from build123d import *

# Parameters (mm, degrees)
F0_W     = 47.752
F0_H     = 16.1036
F1_DEPTH = 5.588
F2_R     = 2.413
F3_DEPTH = 1.8034
F5_W     = 45.212
F5_H     = 13.5636
F5_R     = 3.2512
F6_DEPTH = 9.906


with BuildPart() as f1:
    # F0 (on Top) → F1 (new body, symmetric)
    with BuildSketch(Plane.XY):
        Rectangle(F0_W, F0_H)
    extrude(amount=F1_DEPTH, both=True)

    # F2 (on face) → F3 (join)
    with BuildSketch(Plane.XY.offset(5.588)):
        with Locations((-19.9771, 4.1275)):
            Circle(F2_R)
        with Locations((-12.3571, 4.1275)):
            Circle(F2_R)
        with Locations((-4.7371, 4.1275)):
            Circle(F2_R)
        with Locations((2.8829, 4.1275)):
            Circle(F2_R)
        with Locations((10.5029, 4.1275)):
            Circle(F2_R)
        with Locations((-19.9771, -4.1275)):
            Circle(F2_R)
        with Locations((-12.3571, -4.1275)):
            Circle(F2_R)
        with Locations((-4.7371, -4.1275)):
            Circle(F2_R)
        with Locations((2.8829, -4.1275)):
            Circle(F2_R)
        with Locations((10.5029, -4.1275)):
            Circle(F2_R)
        with Locations((18.1229, 4.1275)):
            Circle(F2_R)
        with Locations((18.1229, -4.1275)):
            Circle(F2_R)
    extrude(amount=F3_DEPTH)

    # F5 (on face) → F6 (cut)
    with BuildSketch(Plane(origin=(0, 0, -5.588), x_dir=(1, 0, 0), z_dir=(0, 0, -1))):
        Rectangle(F5_W, F5_H)
        with Locations((-16.51, 0)):
            Circle(F5_R, mode=Mode.SUBTRACT)
        with Locations((-8.3058, 0)):
            Circle(F5_R, mode=Mode.SUBTRACT)
        with Locations((-0.1016, 0)):
            Circle(F5_R, mode=Mode.SUBTRACT)
        with Locations((8.1026, 0)):
            Circle(F5_R, mode=Mode.SUBTRACT)
        with Locations((16.3068, 0)):
            Circle(F5_R, mode=Mode.SUBTRACT)
    extrude(amount=-F6_DEPTH, mode=Mode.SUBTRACT)


solid = f1.part
Input: part model. Units: mm. Frame: model coordinates. A direction names the side the tool comes from. Coordinates: 2 decimals unless noted, no trailing zeros. Order: outer loops, then holes, each group sorted by start corner. A loop starts at its lowest first (then second) coordinate and runs counter-clockwise, first axis right, second up.
1. Cut plane B-B, the plane y = 0. Return loops of the section in (x, z).
Checked values:
outline: (-23.88, -5.59) - (-22.61, -5.59) - (-22.61, 4.32) - (-19.76, 4.32) - (-19.76, -5.59) - (-13.26, -5.59) - (-13.26, 4.32) - (-11.56, 4.32) - (-11.56, -5.59) - (-5.05, -5.59) - (-5.05, 4.32) - (-3.35, 4.32) - (-3.35, -5.59) - (3.15, -5.59) - (3.15, 4.32) - (4.85, 4.32) - (4.85, -5.59) - (11.35, -5.59) - (11.35, 4.32) - (13.06, 4.32) - (13.06, -5.59) - (19.56, -5.59) - (19.56, 4.32) - (22.61, 4.32) - (22.61, -5.59) - (23.88, -5.59) - (23.88, 5.59) - (-23.88, 5.59) - close
2. Ray query, line 1 along Y through (x, z) = (-21, -4.5); line 2 along X through (y, z) = (-6.25, 3.25); line 3 along Y through (x, z) = (1.5, -2). Return the intervals inside material, ascending.
Checked values:
line 1: y = -8.05 to -6.78, 6.78 to 8.05
line 2: x = -23.88 to -22.61, 22.61 to 23.88
line 3: y = -8.05 to -6.78, -2.83 to 2.83, 6.78 to 8.05
3. Draft query along X for faces 1 (the flat face through (-20, 4, 7.391)), 2 (the cylindrical face through (16.21, -5.6, 6.48)). Return one class per face: +X half, -X half, draft (parallel to the pull), parting line (faces both ways), or undercut.
Checked values:
face 1: draft
face 2: undercut
4. Access query for faces 3 (the cylindrical face through (12.73, 3.2, 6.48)), 4 (the flat face through (0, 6.782, -1)), 5 (the flat face through (-5, -4, 7.391)). Directions: +Z, -Z, +X, -X, +Y, -Y. A direction counts if a zero-diameter tool reaches every point of the face in a straight line with its end or side. Return the directions, or none.
Checked values:
face 3: +Z
face 4: -Z
face 5: +Z, +X, -X, +Y, -Y
5. Cut plane C-C, the plane z = 6.25. Count the separate pieces of the cut face and the enclosed holes in it, plus the area to 3 significant figures.
Checked values:
separate pieces: 12
enclosed holes: 0
area: 220 mm2
6. Cut plane A-A, the plane z = 2.75. Return loops of the section in (x, y).
Checked values:
outline: (-23.88, -8.05) - (23.88, -8.05) - (23.88, 8.05) - (-23.88, 8.05) - close; circle Ø6.5 at (-16.51, 0); circle Ø6.5 at (-8.31, 0); circle Ø6.5 at (-0.1, 0); circle Ø6.5 at (8.1, 0); circle Ø6.5 at (16.31, 0); hole (-22.61, -6.78) - (22.61, -6.78) - (22.61, 6.78) - (-22.61, 6.78) - close
7. Cut plane D-D, the plane x = -16.51. Return loops of the section in (y, z).
Checked values:
outline: (-8.05, -5.59) - (-6.78, -5.59) - (-6.78, 4.32) - (-3.25, 4.32) - (-3.25, -5.59) - (3.25, -5.59) - (3.25, 4.32) - (6.78, 4.32) - (6.78, -5.59) - (8.05, -5.59) - (8.05, 5.59) - (-8.05, 5.59) - close
